from build123d import *

# Parameters (mm, degrees)
BOX003_W        = 6
BOX003_H        = 4
BOX003_DEPTH    = 15
BOX002_W        = 10
BOX002_H        = 10
BOX002_DEPTH    = 15
BOX001_W        = 13
BOX001_H        = 27
BOX001_DEPTH    = 12
BOX_W           = 16
BOX_H           = 40
BOX_DEPTH       = 14
BOX_PITCH_ANGLE = 1.455764


with BuildPart() as cone:
    # Cone → Cone (revolve)
    with BuildSketch(Plane(origin=(8.5, 1, 2), x_dir=(1, 0, 0), z_dir=(0, -1, 0))):
        Polygon((0, 0), (1, 0), (2, 5), (0, 5), align=None)
    revolve(axis=Axis((8.5, 1, 2), (0, 0, 1)))


with BuildPart() as pinhole:
    # Sphere → Sphere (revolve)
    with BuildSketch(Plane(origin=(8.5, 1.25, 7), x_dir=(1, 0, 0), z_dir=(0, -1, 0))):
        with BuildLine():
            ThreePointArc((0, -2.5), (2.5, 0), (0, 2.5))
            Line((0, 2.5), (0, -2.5))
        make_face()
    revolve(axis=Axis((8.5, 1.25, 7), (0, 0, 1)))


with BuildPart() as neck:
    # Box003 → Box003 (new body)
    with BuildSketch(Plane(origin=(5.5, 28, 4), x_dir=(1, 0, 0), z_dir=(0, 0, 1))):
        with Locations((3, 2)):
            Rectangle(BOX003_W, BOX003_H)
    extrude(amount=BOX003_DEPTH)


with BuildPart() as pullbay:
    # Box002 → Box002 (new body)
    with BuildSketch(Plane(origin=(3.5, 30, 2), x_dir=(1, 0, 0), z_dir=(0, 0, 1))):
        with Locations((5, 5)):
            Rectangle(BOX002_W, BOX002_H)
    extrude(amount=BOX002_DEPTH)


with BuildPart() as solenoidbay:
    # Box001 → Box001 (new body)
    with BuildSketch(Plane(origin=(2, 2, 2), x_dir=(1, 0, 0), z_dir=(0, 0, 1))):
        with Locations((6.5, 13.5)):
            Rectangle(BOX001_W, BOX001_H)
    extrude(amount=BOX001_DEPTH)


with BuildPart() as cut004:
    # Box → Box (new body)
    with BuildSketch(Plane.XY):
        with Locations((8, 20)):
            Rectangle(BOX_W, BOX_H)
    extrude(amount=BOX_DEPTH)


with BuildPart() as cut004_1:
    # Box pitch: moved
    add(cut004.part.rotate(Axis((0, 0, 0), (0, 1, 0)), BOX_PITCH_ANGLE))


with BuildPart() as cut004_2:
    # Box placement: moved
    add(cut004_1.part)

    # Cut: cut solenoidBay
    add(solenoidbay.part, mode=Mode.SUBTRACT)

    # Cut001: cut pullBay
    add(pullbay.part, mode=Mode.SUBTRACT)

    # Cut002: cut neck
    add(neck.part, mode=Mode.SUBTRACT)

    # Cut003: cut pinhole
    add(pinhole.part, mode=Mode.SUBTRACT)

    # Cut004: cut Cone
    add(cone.part, mode=Mode.SUBTRACT)


solid = cut004_2.part
Geometry check sheet. Reference: the model listing, model coordinates, mm. A direction names the side the tool comes from. Coordinates: 2 decimals unless noted, no trailing zeros. Order: outer loops, then holes, each group sorted by start corner. A loop starts at its lowest first (then second) coordinate and runs counter-clockwise, first axis right, second up. Notation, with made-up numbers: (-17.5, 83.25) - (-11.5, 83.25) arc R18 ccw to (-11.5, 93.25) - close; hole circle Ø6 at (46, -14.75). An arc over 180 degrees is marked (long way). Answer in a Markdown table with one row per item. Add a question column.
1) Cross-section at D-D, the plane z = 3.5. Record the cut outline in (x, y), then the cut area to 3 significant figures.
2) Gauge pin test, flat ends, axial feed: P1, Ø0.5, axis at x = 7.5, y = 29.5, coming from the +Z side; P2, Ø6.5, axis at x = 6, y = 13, coming from the +Z side; P3, Ø0.5, axis at y = 29.5, z = 7, coming from the +X side. Record the tip position at first contact, or that the pin passes through.
3) Set-up check for faces 4 (the flat face through (3, 40, 5)), 5 (the conical face through (9.76, 0.97, 3.3)), 6 (the flat face through (12, 30, 7)), 7 (the flat face through (9.9, 2, 9.2)): record each of +Z, -Z, +X, -X, +Y, -Y from which the full face is reachable in a straight line by a thin tool's end or side.
4) Release check for a two-part mould opening along X. For faces 1 (the conical face through (7.24, 1.03, 3.3)), 2 (the flat face through (6, 0, 7)), 3 (the flat face through (3.5, 35, 8)) record: +X half, -X half, draft (parallel to the pull), parting line (faces both ways), or undercut.
5) Cross-section at C-C, the plane z = 6.25. Record the cut outline in (x, y), then the cut area to 3 significant figures.
6) Cross-section at A-A, the plane y = 4. Record the cut outline in (x, z), then the cut area to 3 significant figures.
7) Cross-section at B-B, the plane z = 8. Record the cut outline in (x, y).
8) Material ranges on line 1 along Y through (x, z) = (12.75, 4.75); line 2 along Y through (x, z) = (14, 10.75); line 3 along Y through (x, z) = (8.75, 13), recorded low to high. Write a range as [from, to].
Check result:
| question | item | result |
|---|---|---|
| 1 | outline | (0.09, 0) - (7.67, 0) arc R1.3 cw to (7.67, 2) - (2, 2) - (2, 29) - (15, 29) - (15, 2) - (9.33, 2) arc R1.3 cw to (9.33, 0) - (16.09, 0) - (16.09, 40) - (13.5, 40) - (13.5, 30) - (3.5, 30) - (3.5, 40) - (0.09, 40) - close |
| 1 | area | 185 mm² |
| 2 | P1 | stops at z = 4 |
| 2 | P2 | stops at z = 2 |
| 2 | P3 | stops at x = 16.19 |
| 3 | face 4 | +Z, -Z, +X, -X, +Y |
| 3 | face 5 | none |
| 3 | face 6 | +Z, +Y |
| 3 | face 7 | +Z |
| 4 | face 1 | undercut |
| 4 | face 2 | draft |
| 4 | face 3 | undercut |
| 5 | outline | (0.16, 0) - (6.47, 0) arc R2.38 cw to (6.24, 2) - (2, 2) - (2, 29) - (5.5, 29) - (5.5, 30) - (3.5, 30) - (3.5, 40) - (0.16, 40) - close; (10.53, 0) - (16.16, 0) - (16.16, 40) - (13.5, 40) - (13.5, 30) - (11.5, 30) - (11.5, 29) - (15, 29) - (15, 2) - (10.76, 2) arc R2.38 cw to start |
| 5 | area | 174 mm² |
| 6 | outline | (0, 0) - (15.99, -0.41) - (16.35, 13.59) - (15, 13.62) - (15, 2) - (2, 2) - (2, 13.95) - (0.36, 14) - close |
| 6 | area | 70.7 mm² |
| 7 | outline | (0.2, 0) - (6.58, 0) arc R2.29 cw to (6.33, 2) - (2, 2) - (2, 29) - (5.5, 29) - (5.5, 30) - (3.5, 30) - (3.5, 40) - (0.2, 40) - close; (10.42, 0) - (16.21, 0) - (16.21, 40) - (13.5, 40) - (13.5, 30) - (11.5, 30) - (11.5, 29) - (15, 29) - (15, 2) - (10.67, 2) arc R2.29 cw to start |
| 8 | line 1 | y = [0, 2], [29, 30] |
| 8 | line 2 | y = [0, 2], [29, 40] |
| 8 | line 3 | y = [0, 2] |
